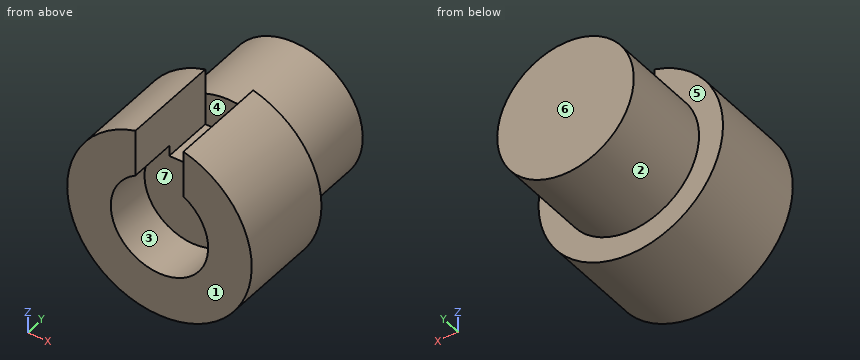
from build123d import *

# Parameters (mm, degrees)
SKETCH_1_R          = 4.275
EXTRUDE_1_DEPTH     = 12
SKETCH_3_R          = 5.775
EXTRUDE_2_DEPTH     = 6.2
SKETCH_2_R          = 3.05
CUT_EXTRUDE_1_DEPTH = 3
SKETCH_4_W          = 3
SKETCH_4_H          = 6.2
CUT_EXTRUDE_2_DEPTH = 4


with BuildPart() as part:
    # 草图1 → 凸台-拉伸1 (new body)
    with BuildSketch(Plane(origin=(0, 0, 0), x_dir=(1, 0, 0), z_dir=(0, 1, 0))):
        with Locations(Location((0, 0, 0), (0, 0, 270))):
            Circle(SKETCH_1_R)
    extrude(amount=EXTRUDE_1_DEPTH)

    # 草图3 → 凸台-拉伸2 (add)
    with BuildSketch(Plane.XZ):
        with Locations(Location((0, 0, 0), (0, 0, 270))):
            Circle(SKETCH_3_R)
    extrude(amount=-EXTRUDE_2_DEPTH)

    # 草图2 → 切除-拉伸1 (cut)
    with BuildSketch(Plane.XZ):
        with Locations(Location((0, 0, 0), (0, 0, 270))):
            Circle(SKETCH_2_R)
    extrude(amount=-CUT_EXTRUDE_1_DEPTH, mode=Mode.SUBTRACT)

    # 草图4 → 切除-拉伸2 (cut)
    with BuildSketch(Plane.XY.offset(6)):
        with Locations((0, 3.1)):
            Rectangle(SKETCH_4_W, SKETCH_4_H)
    extrude(amount=-CUT_EXTRUDE_2_DEPTH, mode=Mode.SUBTRACT)


solid = part.part
Verification items for the finished model (mm, model axes). Face numbers are marked on the shaded views. A direction names the side the tool comes from. Coordinates: 2 decimals unless noted, no trailing zeros. Order: outer loops, then holes, each group sorted by start corner. A loop starts at its lowest first (then second) coordinate and runs counter-clockwise, first axis right, second up. Notation, with made-up numbers: M 63,86.5 L 78,86.5 A15 ccw 78,104.5 Z; hole C -26,-7 d11. An arc over 180 degrees is marked long. One line per item, written item: value. Start each with the question number.
Item 1: Scan lines: probe 1 along X at (y, z) = (0.85, 0) (3 decimals); probe 2 along Z at (x, y) = (0, 1.65) (3 decimals); probe 3 along Y at (x, z) = (-2.25, 4). Record each from-to range of solid material in increasing order.
Item 2: Mould release check, pull along X, two halves, no side actions. Record for the marked faces 1, 2 and 3: released by +X, released by -X, zero draft, split by the parting line, or undercut.
Item 3: Gauge pin test, flat ends, axial feed: pin 1 (1.1 mm diameter, centred on y = 3.5, z = 4, fed in from -X); pin 2 (1 mm diameter, centred on y = 5, z = 3.5, fed in from -X); pin 3 (3 mm diameter, centred on x = -0.5, z = -0.5, fed in from -Y); pin 4 (6 mm diameter, centred on y = 6.5, z = -2, fed in from +X) (3 decimals). Record the tip position at first contact, or that the pin passes through.
Item 4: Sectioned sample at D-D (x = -3.75). Enter the section's corners in (y, z).
Item 5: Sectioned sample at C-C (y = 4.75). Enter the section's corners in (x, z) (3 decimals).
Item 6: Sectioned sample at B-B (z = 0). Enter the section's corners in (x, y) (3 decimals), then the cut area to 3 significant figures.
Item 7: Access from +Z, -Z, +X, -X, +Y, -Y to the whole of each face (thin tool, end or side, straight path). Record for the marked faces 4, 5, 6 and 7.
Item 8: Sectioned sample at A-A (x = -1). Enter the section's corners in (y, z), then the cut area to 3 significant figures.
Conclusion:
1. probe 1: x = -5.775 to -3.05, 3.05 to 5.775
1. probe 2: z = -5.775 to -3.05
1. probe 3: y = 0 to 6.2
2. face 1: zero draft
2. face 2: split by the parting line
2. face 3: undercut
3. pin 1: stops at x = -4.63
3. pin 2: stops at x = -4.93
3. pin 3: stops at y = 3
3. pin 4: stops at x = 5.775
4. outline: M 0,-4.39 L 6.2,-4.39 L 6.2,-2.05 L 12,-2.05 L 12,2.05 L 6.2,2.05 L 6.2,4.39 L 0,4.39 Z
5. outline: M -1.5,2 L -1.5,5.577 A5.775 ccw long 1.5,5.577 L 1.5,2 Z
6. outline: M -5.775,0 L -3.05,0 L -3.05,3 L 3.05,3 L 3.05,0 L 5.775,0 L 5.775,6.2 L 4.275,6.2 L 4.275,12 L -4.275,12 L -4.275,6.2 L -5.775,6.2 Z
6. area: 103 mm^2
7. face 4: +Z, -Y
7. face 5: +Y
7. face 6: +Z, -Z, +X, -X, +Y
7. face 7: -Y
8. outline: M 0,-5.69 L 6.2,-5.69 L 6.2,-4.16 L 12,-4.16 L 12,4.16 L 6.2,4.16 L 6.2,2 L 3,2 L 3,-2.88 L 0,-2.88 Z
8. area: 81.2 mm^2
